```python
from build123d import *

# Parameters (mm, degrees)
ESQUISSE1_R             = 11
BOSS_EXTRU_2_DEPTH      = 5
ESQUISSE3_W             = 50
ESQUISSE3_H             = 5
BOSS_EXTRU_4_DEPTH      = 5
ESQUISSE2_W             = 50
ESQUISSE2_H             = 5
BOSS_EXTRU_3_DEPTH      = 45
ESQUISSE4_R             = 1.5
ENL_V_MAT_EXTRU_1_DEPTH = 60.581876439
CONG_1_R                = 5
ESQUISSE5_R             = 1.5
ESQUISSE5_R_2           = 11
BOSS_EXTRU_5_DEPTH      = 5
BOSS_EXTRU_6_START      = -0.5
BOSS_EXTRU_6_DEPTH      = 3
ESQUISSE9_R             = 2
ENL_V_MAT_EXTRU_3_DEPTH = 106.948100502


with BuildPart() as part:
    # Esquisse1 → Boss.-Extru.2 (new body)
    with BuildSketch(Plane.XY):
        with BuildLine():
            Line((-20, 25), (20, 25))
            ThreePointArc((20, 25), (23.535533906, 23.535533906), (25, 20))
            Line((25, 20), (25, -25))
            Line((25, -25), (-25, -25))
            Line((-25, -25), (-25, 20))
            ThreePointArc((-25, 20), (-23.535533906, 23.535533906), (-20, 25))
        make_face()
        Circle(ESQUISSE1_R, mode=Mode.SUBTRACT)
    extrude(amount=BOSS_EXTRU_2_DEPTH)

    # Esquisse3 → Boss.-Extru.4 (add)
    with BuildSketch(Plane.XZ.offset(25)):
        with Locations((0, 2.5)):
            Rectangle(ESQUISSE3_W, ESQUISSE3_H)
    extrude(amount=BOSS_EXTRU_4_DEPTH)

    # Esquisse2 → Boss.-Extru.3 (add)
    with BuildSketch(Plane.XY.offset(5)):
        with Locations((0, -27.5)):
            Rectangle(ESQUISSE2_W, ESQUISSE2_H)
    extrude(amount=BOSS_EXTRU_3_DEPTH)

    # Esquisse4 → Enlèv. mat.-Extru.1 (cut, through all)
    with BuildSketch(Plane.XY.offset(5)):
        with Locations((-15.5, 15.5)):
            Circle(ESQUISSE4_R)
        with Locations((15.5, 15.5)):
            Circle(ESQUISSE4_R)
        with Locations((15.5, -15.5)):
            Circle(ESQUISSE4_R)
        with Locations((-15.5, -15.5)):
            Circle(ESQUISSE4_R)
    extrude(amount=-ENL_V_MAT_EXTRU_1_DEPTH, mode=Mode.SUBTRACT)

    # Congé1
    cong_1_edges = [part.edges().sort_by_distance(p)[0] for p in [
        (25, -27.5, 50),
        (-25, -27.5, 50),
    ]]
    fillet(cong_1_edges, radius=CONG_1_R)

    # Esquisse5 → Boss.-Extru.5 (add)
    # profile 1 of 3: a face of its own
    with BuildSketch(Plane(origin=(0, 0, 0), x_dir=(-1, 0, 0), z_dir=(0, 0, -1))):
        with BuildLine():
            ThreePointArc((-20, 25), (-23.535533906, 23.535533906), (-25, 20))
            Line((-25, 20), (-25, -30))
            Line((-25, -30), (25, -30))
            Line((25, -30), (25, 20))
            ThreePointArc((25, 20), (23.535533906, 23.535533906), (20, 25))
            Line((20, 25), (-20, 25))
        make_face()
        with Locations(Location((-15.5, -15.5, 0), (0, 0, 180))):
            Circle(ESQUISSE5_R, mode=Mode.SUBTRACT)
        with Locations(Location((-15.5, 15.5, 0), (0, 0, 180))):
            Circle(ESQUISSE5_R, mode=Mode.SUBTRACT)
        with Locations(Location((0, 0, 0), (0, 0, 180))):
            Circle(ESQUISSE5_R_2, mode=Mode.SUBTRACT)
        with Locations(Location((15.5, -15.5, 0), (0, 0, 180))):
            Circle(ESQUISSE5_R, mode=Mode.SUBTRACT)
        with Locations(Location((15.5, 15.5, 0), (0, 0, 180))):
            Circle(ESQUISSE5_R, mode=Mode.SUBTRACT)
    # profile 2 of 3: a face of its own
    with BuildSketch(Plane(origin=(0, 0, 0), x_dir=(-1, 0, 0), z_dir=(0, 0, -1))):
        with BuildLine():
            Line((-25, 55), (-25, 20))
            ThreePointArc((-25, 20), (-23.535533906, 23.535533906), (-20, 25))
            Line((-20, 25), (20, 25))
            ThreePointArc((20, 25), (23.535533906, 23.535533906), (25, 20))
            Line((25, 20), (25, 55))
            ThreePointArc((25, 55), (22.071067812, 62.071067812), (15, 65))
            Line((15, 65), (-15, 65))
            ThreePointArc((-15, 65), (-22.071067812, 62.071067812), (-25, 55))
        make_face()
        with Locations((0, 60)):
            Circle(ESQUISSE5_R, mode=Mode.SUBTRACT)
    # profile 3 of 3: a face of its own
    with BuildSketch(Plane(origin=(0, 0, 0), x_dir=(-1, 0, 0), z_dir=(0, 0, -1))):
        with BuildLine():
            ThreePointArc((-20, 25), (-23.535533906, 23.535533906), (-25, 20))
            Line((-25, 20), (-25, -30))
            Line((-25, -30), (25, -30))
            Line((25, -30), (25, 20))
            ThreePointArc((25, 20), (23.535533906, 23.535533906), (20, 25))
            Line((20, 25), (-20, 25))
        make_face()
        with Locations(Location((-15.5, -15.5, 0), (0, 0, 180))):
            Circle(ESQUISSE5_R, mode=Mode.SUBTRACT)
        with Locations(Location((-15.5, 15.5, 0), (0, 0, 180))):
            Circle(ESQUISSE5_R, mode=Mode.SUBTRACT)
        with Locations(Location((0, 0, 0), (0, 0, 180))):
            Circle(ESQUISSE5_R_2, mode=Mode.SUBTRACT)
        with Locations(Location((15.5, -15.5, 0), (0, 0, 180))):
            Circle(ESQUISSE5_R, mode=Mode.SUBTRACT)
        with Locations(Location((15.5, 15.5, 0), (0, 0, 180))):
            Circle(ESQUISSE5_R, mode=Mode.SUBTRACT)
    extrude(amount=-BOSS_EXTRU_5_DEPTH)

    # Esquisse7 → Boss.-Extru.6 (add)
    with BuildSketch(Plane.ZY.offset(25).offset(BOSS_EXTRU_6_START)):
        Polygon((25, -25), (5, 35), (5, -25), align=None)
    boss_extru_6 = extrude(amount=-BOSS_EXTRU_6_DEPTH)

    # Symétrie1: Boss.-Extru.6 across plane
    add(boss_extru_6.mirror(Plane(origin=(0, 0, 0), x_dir=(0, 0, 1), z_dir=(1, 0, 0))))

    # Esquisse9 → Enlèv. mat.-Extru.3 (cut, through all)
    with BuildSketch(Plane(origin=(0, -25, 0), x_dir=(1, 0, 0), z_dir=(0, 1, 0))):
        with Locations(Location((-15, -35, 0), (0, 0, 270))):
            Circle(ESQUISSE9_R)
        with Locations(Location((15, -35, 0), (0, 0, 90))):
            Circle(ESQUISSE9_R)
        with Locations(Location((0, -17.5, 0), (0, 0, 270))):
            Circle(ESQUISSE9_R)
    extrude(amount=-ENL_V_MAT_EXTRU_3_DEPTH, mode=Mode.SUBTRACT)


solid = part.part
```
Verification items for the finished model (mm, model axes). A direction names the side the tool comes from. Coordinates: 2 decimals unless noted, no trailing zeros. Loops run counter-clockwise (first coordinate to the right, second up) from the corner with the lowest first, then second, coordinate; pieces in that order, holes last. Notation, with made-up numbers: (75.25, 67) - (126.25, 67) arc R15 cw to (126.25, 71) - close; hole circle Ø11 at (43.5, -7.75). An arc over 180 degrees is marked (long way). Return JSON: item names as keys, results as strings.
1. Section check B-B, the plane y = 15.5. Record the boundary of the cut face in (x, z), then the cut area to 3 significant figures.
Established:
{"outline": "(-25, 0) - (-17, 0) - (-17, 5) - (-21.5, 5) - (-21.5, 11.5) - (-24.5, 11.5) - (-24.5, 5) - (-25, 5) - close; (-14, 0) - (14, 0) - (14, 5) - (-14, 5) - close; (17, 0) - (25, 0) - (25, 5) - (24.5, 5) - (24.5, 11.5) - (21.5, 11.5) - (21.5, 5) - (17, 5) - close", "area": "259 mm2"}
2. Section check C-C, the plane x = -6.5. Record the boundary of the cut face in (y, z), then the cut area to 3 significant figures.
Established:
{"outline": "(-30, 0) - (-8.87, 0) - (-8.87, 5) - (-25, 5) - (-25, 50) - (-30, 50) - close; (8.87, 0) - (65, 0) - (65, 5) - (8.87, 5) - close", "area": "611 mm2"}
3. Thickness scan on L1, parallel to X at y = -28, z = 35; L2, parallel to Y at x = 0, z = 3.55; L3, parallel to X at y = 18, z = 10. Record the ranges inside material, lowest first.
Established:
{"L1": "x = -25 to -17, -13 to 13, 17 to 25", "L2": "y = -30 to -11, 11 to 58.5, 61.5 to 65", "L3": "x = -24.5 to -21.5, 21.5 to 24.5"}
4. Tool access check on faces 4 (the flat face through (-24.5, -8, 10)), 5 (the flat face through (0, 21, 5)), 6 (the flat face through (23, 5, 15)). Record the directions out of +Z, -Z, +X, -X, +Y, -Y that give a thin tool (end or side, any length) a straight path to the whole face; none if there is none.
Established:
{"face 4": "+Z, -X, +Y", "face 5": "+Z, +Y", "face 6": "+Z, +X, -X, +Y"}
5. Section check A-A, the plane z = 35. Record the boundary of the cut face in (x, y).
Established:
{"outline": "(-25, -30) - (-17, -30) - (-17, -25) - (-25, -25) - close; (-13, -30) - (13, -30) - (13, -25) - (-13, -25) - close; (17, -30) - (25, -30) - (25, -25) - (17, -25) - close"}
6. Mould release check, pull along Y, two halves, no side actions. Record for faces 1 (the flat face through (21.5, -8, 10)), 2 (the flat face through (0, 65, 2)), 3 (the cylindrical face through (-17, -15.43, 2.54)): +Y half, -Y half, draft (parallel to the pull), parting line (faces both ways), or undercut.
Established:
{"face 1": "draft", "face 2": "+Y half", "face 3": "undercut"}
7. Go/stop test with flat-tipped pins: pin 1 (5 mm diameter, centred on x = 15.5, y = 15.5, fed in from +Z); pin 2 (8 mm diameter, centred on x = -12, z = 35.5, fed in from +Y); pin 3 (6 mm diameter, centred on y = 12, z = 12.5, fed in from -X). Record where each tip stops, or that it passes through.
Established:
{"pin 1": "stops at z = 5", "pin 2": "stops at y = -25", "pin 3": "stops at x = -24.5"}
8. Section check D-D, the plane y = 0. Record the boundary of the cut face in (x, z).
Established:
{"outline": "(-25, 0) - (-11, 0) - (-11, 5) - (-21.5, 5) - (-21.5, 16.67) - (-24.5, 16.67) - (-24.5, 5) - (-25, 5) - close; (11, 0) - (25, 0) - (25, 5) - (24.5, 5) - (24.5, 16.67) - (21.5, 16.67) - (21.5, 5) - (11, 5) - close"}
